Solid Edge part; units mm, degrees
sketch "Sketch1" plane through (0, 0, 0) normal (0, 0, 1) x (1, 0, 0)
  circle A0 centre (0, 0) radius 40
extrude "Protrusion1" add sketch "Sketch1" along normal blind 60
sketch "Sketch2" plane through (0, 0, 60) normal (0, 0, 1) x (0, 1, 0)
  line L0 (10, -5) -> (-10, -5)
  line L1 (-10, -5) -> (-10, 5)
  line L2 (-10, 5) -> (10, 5)
  line L3 (10, 5) -> (10, -5)
extrude "ProtrusiónExtruida_2" add sketch "Sketch2" along normal blind 28
sketch "Sketch3" plane through (5, 0, 74) normal (1, 0, 0) x (0, 1, 0)
  circle A0 centre (0, 4) radius 2.5
extrude "Cutout1" cut sketch "Sketch3" against normal up to next
fillet "Redondeo_1" radius 10 4 edges at (0, -10, 88) (0, 10, 88) (0, -10, 60) (0, 10, 60)
sketch "Sketch4" plane through (0, 0, 0) normal (0, 0, -1) x (0, 1, 0)
  circle A0 centre (0, 0) radius 2.5
extrude "VaciadoExtruido_2" cut sketch "Sketch4" against normal blind 30
sketch "Sketch5" plane through (0, 0, 60) normal (0, 0, 1) x (0, 1, 0)
  line L0 (-40, -40) -> (40, -40)
  line L1 (40, -40) -> (40, -30)
  line L2 (40, -30) -> (-40, -30)
  line L3 (-40, -30) -> (-40, -40)
extrude "Cutout2" cut sketch "Sketch5" against normal through all
chamfer "Chaflán_1" distance 2 angle 45 2 edges at (-40, 0, 60) (30, 0, 60)
CAD build for the part. Positions are in the model's coordinates, mm. A direction names the side the tool comes from. Round coordinates to 2 decimals unless told otherwise and drop trailing zeros. Order: outer loops, then holes, each group sorted by start corner. A loop starts at its lowest first (then second) coordinate and runs counter-clockwise, first axis right, second up. Notation, with made-up numbers: (-17, 46.5) -> (5, 46.5) arc R35 cw to (5, 80.5) -> close; hole circle Ø6 at (11, 59). An arc over 180 degrees is marked (long way). Write item = value, one per line.
(1) Pull direction X, two halves, no side cores. Call faces 6 (the flat face through (30, 0, 29)), 7 (the flat face through (0, 0, 30)), 8 (the cylindrical face through (0.07, 7.15, 84.99)), 9 (the cylindrical face through (-39.977, -1.354, 28.594)): +X half, -X half, draft (parallel to the pull), parting line (faces both ways), or undercut.
Answers follow:
face_6 = +X half
face_7 = undercut
face_8 = draft
face_9 = parting line
(2) 3-axis set-ups, long thin cutter, end or side, ignore diameter. For faces 1 (the cylindrical face through (-2.44, -0.54, 14.79)), 2 (the flat face through (5, 0, 71)), 3 (the flat face through (-5, 0, 71)), 4 (the flat face through (0, -10, 74)), 5 (the flat face through (0, 10, 74)): which of +Z, -Z, +X, -X, +Y, -Y reach the whole face in a straight line?
Answers follow:
face_1 = -Z
face_2 = +Z, +X, +Y, -Y
face_3 = +Z, -X, +Y, -Y
face_4 = +Z, +X, -X, -Y
face_5 = +Z, +X, -X, +Y
(3) Cut at C-C (z = 37.5). Write the cut outline in (x, y).
Answers follow:
outline = (30, -26.46) -> (30, 26.46) arc R40 ccw (long way) to start
(4) Drill centre lines: L1, parallel to Z at x = 2.75, y = 0; L2, parallel to Z at x = 0.75, y = 0; L3, parallel to Z at x = 12, y = -14.5. Where is each one in solid material? Low to high.
Answers follow:
L1 = 0 to 75.5, 80.5 to 88
L2 = 30 to 75.5, 80.5 to 88
L3 = 0 to 60
(5) Flat gauge pins, fed straight in: P1, Ø2.5, axis at x = 0.5, y = -1, coming from the -Z side; P2, Ø9, axis at x = 0.5, z = 73, coming from the +Y side; P3, Ø8, axis at x = -21, z = 18.5, coming from the +Y side; P4, Ø4.5, axis at y = 0, z = 78, coming from the -X side. Where does each tip first touch, or does it go through?
Answers follow:
P1 = 30
P2 = 10.11
P3 = 36.21
P4 = through
(6) Cut at B-B (z = 28.5). Write the cut outline in (x, y).
Answers follow:
outline = (30, -26.46) -> (30, 26.46) arc R40 ccw (long way) to start; hole circle Ø5 at (0, 0)
